CAD build for the part. Positions are in the model's coordinates, mm. Round coordinates to 2 decimals unless told otherwise and drop trailing zeros. Loops run counter-clockwise (first coordinate to the right, second up) from the corner with the lowest first, then second, coordinate; pieces in that order, holes last. Notation, with made-up numbers: (-36.75, 74.25) - (-3.75, 74.25) arc R18 ccw to (-3.75, 105.25) - close; hole circle Ø3 at (-21.75, 77). An arc over 180 degrees is marked (long way). Use one line per item in the form item = value.
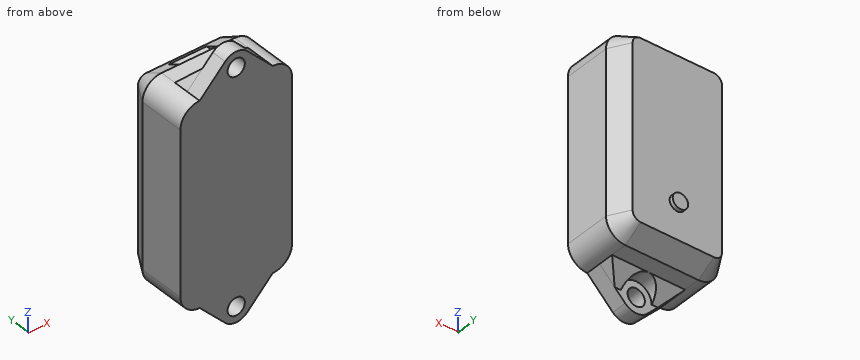
from build123d import *
from OCP.BRepFilletAPI import BRepFilletAPI_MakeChamfer

# Parameters (mm, degrees)
Y_KSEKLIK_EKSTR_ZYON2_DEPTH = 17.25
IZIM1_3_R                   = 2.25
Y_KSEKLIK_EKSTR_ZYON3_DEPTH = 4
PAH2_SIZE                   = 5
PAH2_SIZE2                  = 2.886751346
Y_KSEKLIK_EKSTR_ZYON4_DEPTH = 4
KES_EKSTR_ZYON2_DEPTH       = 24
IZIM7_W                     = 10
IZIM7_H                     = 2
KES_EKSTR_ZYON3_DEPTH       = 5
IZIM8_R                     = 2
Y_KSEKLIK_EKSTR_ZYON6_DEPTH = 1
IZIM10_R                    = 4
KES_EKSTR_ZYON4_DEPTH       = 10
IZIM11_R                    = 4
KES_EKSTR_ZYON5_DEPTH       = 10
KES_EKSTR_ZYON6_DEPTH       = 30


with BuildPart() as part:
    # izim1 → Y_kseklik-Ekstr_zyon2 (new body)
    with BuildSketch(Plane(origin=(0, 0, 0), x_dir=(1, 0, 0), z_dir=(0, 1, 0))):
        with BuildLine():
            Line((0, 26), (0, 5))
            ThreePointArc((0, 5), (1.464466094, 1.464466094), (5, 0))
            Line((5, 0), (24, 0))
            ThreePointArc((24, 0), (27.535533906, 1.464466094), (29, 5))
            Line((29, 5), (29, 26))
            Line((29, 26), (0, 26))
        make_face()
        with BuildLine():
            Line((0, 47), (0, 26))
            Line((0, 26), (29, 26))
            Line((29, 26), (29, 47))
            ThreePointArc((29, 47), (27.535533906, 50.535533906), (24, 52))
            Line((24, 52), (5, 52))
            ThreePointArc((5, 52), (1.464466094, 50.535533906), (0, 47))
        make_face()
    extrude(amount=Y_KSEKLIK_EKSTR_ZYON2_DEPTH)

    # izim1_3 → Y_kseklik-Ekstr_zyon3 (add)
    # profile 1 of 2: a face of its own
    with BuildSketch(Plane(origin=(0, 0, 0), x_dir=(1, 0, 0), z_dir=(0, 1, 0))):
        with BuildLine():
            ThreePointArc((11.638823529, 58.795294118), (14.5, 60), (17.361176471, 58.795294118))
            Line((17.361176471, 58.795294118), (24, 52))
            Line((24, 52), (5, 52))
            Line((5, 52), (11.638823529, 58.795294118))
        make_face()
        with Locations(Location((14.5, 56, 0), (0, 0, 270))):
            Circle(IZIM1_3_R, mode=Mode.SUBTRACT)
    # profile 2 of 2: a face of its own
    with BuildSketch(Plane(origin=(0, 0, 0), x_dir=(1, 0, 0), z_dir=(0, 1, 0))):
        with BuildLine():
            Line((5, 0), (11.638823529, -6.795294118))
            ThreePointArc((11.638823529, -6.795294118), (14.5, -8), (17.361176471, -6.795294118))
            Line((17.361176471, -6.795294118), (24, 0))
            Line((24, 0), (5, 0))
        make_face()
        with Locations(Location((14.5, -4, 0), (0, 0, 270))):
            Circle(IZIM1_3_R, mode=Mode.SUBTRACT)
    extrude(amount=Y_KSEKLIK_EKSTR_ZYON3_DEPTH)

    # Pah2: one chamfer whose edges measure the first distance from different faces: ONE call of the kernel's chamfer builder (chamfer() names one face for all edges)
    pah2_edges_1 = [part.edges().sort_by_distance(p)[0] for p in [
        (27.535533906, 17.25, -50.535533906),
    ]]
    pah2_side_1 = [part.faces().sort_by_distance(p)[0] for p in [
        (27.535533906, 8.625, -50.535533906),
    ]]
    pah2_edges_2 = [part.edges().sort_by_distance(p)[0] for p in [
        (14.5, 17.25, -52),
    ]]
    pah2_side_2 = [part.faces().sort_by_distance(p)[0] for p in [
        (14.5, 10.625, -52),
    ]]
    pah2_edges_3 = [part.edges().sort_by_distance(p)[0] for p in [
        (1.464466094, 17.25, -50.535533906),
    ]]
    pah2_side_3 = [part.faces().sort_by_distance(p)[0] for p in [
        (1.464466094, 8.625, -50.535533906),
    ]]
    pah2_edges_4 = [part.edges().sort_by_distance(p)[0] for p in [
        (0, 17.25, -26),
    ]]
    pah2_side_4 = [part.faces().sort_by_distance(p)[0] for p in [
        (0, 8.625, -26),
    ]]
    pah2_edges_5 = [part.edges().sort_by_distance(p)[0] for p in [
        (1.464466094, 17.25, -1.464466094),
    ]]
    pah2_side_5 = [part.faces().sort_by_distance(p)[0] for p in [
        (1.464466094, 8.625, -1.464466094),
    ]]
    pah2_edges_6 = [part.edges().sort_by_distance(p)[0] for p in [
        (14.5, 17.25, 0),
    ]]
    pah2_side_6 = [part.faces().sort_by_distance(p)[0] for p in [
        (14.5, 10.625, 0),
    ]]
    pah2_edges_7 = [part.edges().sort_by_distance(p)[0] for p in [
        (27.535533906, 17.25, -1.464466094),
    ]]
    pah2_side_7 = [part.faces().sort_by_distance(p)[0] for p in [
        (27.535533906, 8.625, -1.464466094),
    ]]
    pah2_edges_8 = [part.edges().sort_by_distance(p)[0] for p in [
        (29, 17.25, -26),
    ]]
    pah2_side_8 = [part.faces().sort_by_distance(p)[0] for p in [
        (29, 8.625, -26),
    ]]
    pah2 = BRepFilletAPI_MakeChamfer(part.part.solid().wrapped)
    for e in pah2_edges_1:
        pah2.Add(PAH2_SIZE, PAH2_SIZE2, e.wrapped, pah2_side_1[0].wrapped)  # the first distance lies on this face
    for e in pah2_edges_2:
        pah2.Add(PAH2_SIZE, PAH2_SIZE2, e.wrapped, pah2_side_2[0].wrapped)  # the first distance lies on this face
    for e in pah2_edges_3:
        pah2.Add(PAH2_SIZE, PAH2_SIZE2, e.wrapped, pah2_side_3[0].wrapped)  # the first distance lies on this face
    for e in pah2_edges_4:
        pah2.Add(PAH2_SIZE, PAH2_SIZE2, e.wrapped, pah2_side_4[0].wrapped)  # the first distance lies on this face
    for e in pah2_edges_5:
        pah2.Add(PAH2_SIZE, PAH2_SIZE2, e.wrapped, pah2_side_5[0].wrapped)  # the first distance lies on this face
    for e in pah2_edges_6:
        pah2.Add(PAH2_SIZE, PAH2_SIZE2, e.wrapped, pah2_side_6[0].wrapped)  # the first distance lies on this face
    for e in pah2_edges_7:
        pah2.Add(PAH2_SIZE, PAH2_SIZE2, e.wrapped, pah2_side_7[0].wrapped)  # the first distance lies on this face
    for e in pah2_edges_8:
        pah2.Add(PAH2_SIZE, PAH2_SIZE2, e.wrapped, pah2_side_8[0].wrapped)  # the first distance lies on this face
    add(Compound.cast(pah2.Shape()), mode=Mode.REPLACE)

    # izim4 → Y_kseklik-Ekstr_zyon4 (add)
    with BuildSketch(Plane(origin=(0, 4, 0), x_dir=(1, 0, 0), z_dir=(0, 1, 0))):
        with BuildLine():
            Line((8.907894737, 56), (12.25, 56))
            ThreePointArc((12.25, 56), (14.5, 53.75), (16.75, 56))
            Line((16.75, 56), (20.092105263, 56))
            Line((20.092105263, 56), (24, 52))
            Line((24, 52), (5, 52))
            Line((5, 52), (8.907894737, 56))
        make_face()
        with BuildLine():
            Line((5, 0), (8.907894737, -4))
            Line((8.907894737, -4), (12.25, -4))
            ThreePointArc((12.25, -4), (14.5, -1.75), (16.75, -4))
            Line((16.75, -4), (20.092105263, -4))
            Line((20.092105263, -4), (24, 0))
            Line((24, 0), (5, 0))
        make_face()
    extrude(amount=Y_KSEKLIK_EKSTR_ZYON4_DEPTH)

    # izim5 → Kes-Ekstr_zyon2 (cut)
    with BuildSketch(Plane.ZY):
        Polygon((0, 8), (4, 4), (4, 8), align=None)
    extrude(amount=-KES_EKSTR_ZYON2_DEPTH, mode=Mode.SUBTRACT)

    # izim7 → Kes-Ekstr_zyon3 (cut)
    with BuildSketch(Plane(origin=(0, 17.25, 0), x_dir=(1, 0, 0), z_dir=(0, 1, 0))):
        with Locations((14.5, 1)):
            Rectangle(IZIM7_W, IZIM7_H)
    extrude(amount=-KES_EKSTR_ZYON3_DEPTH, mode=Mode.SUBTRACT)

    # izim8 → Y_kseklik-Ekstr_zyon6 (add)
    with BuildSketch(Plane(origin=(0, 17.25, 0), x_dir=(1, 0, 0), z_dir=(0, 1, 0))):
        with Locations(Location((14.5, 40, 0), (0, 0, 270))):
            Circle(IZIM8_R)
    extrude(amount=Y_KSEKLIK_EKSTR_ZYON6_DEPTH)

    # izim10 → Kes-Ekstr_zyon4 (cut)
    with BuildSketch(Plane(origin=(0, 4, 0), x_dir=(1, 0, 0), z_dir=(0, 1, 0))):
        with Locations((14.5, 56)):
            Circle(IZIM10_R)
    extrude(amount=KES_EKSTR_ZYON4_DEPTH, mode=Mode.SUBTRACT)

    # izim11 → Kes-Ekstr_zyon5 (cut)
    with BuildSketch(Plane(origin=(0, 4, 0), x_dir=(1, 0, 0), z_dir=(0, 1, 0))):
        with Locations((14.5, -4)):
            Circle(IZIM11_R)
    extrude(amount=KES_EKSTR_ZYON5_DEPTH, mode=Mode.SUBTRACT)

    # izim12 → Kes-Ekstr_zyon6 (cut)
    with BuildSketch(Plane.ZY):
        Polygon((-52, 8), (-56, 8), (-56, 4), align=None)
    extrude(amount=-KES_EKSTR_ZYON6_DEPTH, mode=Mode.SUBTRACT)


solid = part.part
1) Slice it at A-A (z = -40). Write the cut outline in (x, y), plus the area to 3 significant figures.
Report:
outline = (0, 0) - (29, 0) - (29, 12.25) - (26.11, 17.25) - (16.5, 17.25) - (16.5, 18.25) - (12.5, 18.25) - (12.5, 17.25) - (2.89, 17.25) - (0, 12.25) - close
area = 490 mm^2
2) Drill centre lines: probe 1 along X at (y, z) = (2.6, -56); probe 2 along Y at (x, z) = (24.5, -17); probe 3 along Z at (x, y) = (13.5, 2). Where is each one in solid material? Low to high.
Report:
probe_1 = 8.91 to 12.25, 16.75 to 20.09
probe_2 = 0 to 17.25
probe_3 = -59.87 to -58.02, -53.98 to 1.98, 6.02 to 7.87
3) Slice it at B-B (x = 15.5). Write the cut outline in (y, z), plus the area to 3 significant figures.
Report:
outline = (0, -59.87) - (4, -59.87) - (4, -58.02) - (0, -58.02) - close; (0, -53.98) - (4, -53.98) - (4, -52.13) - (7.87, -52.13) - (8, -52) - (12.25, -52) - (17.25, -49.11) - (17.25, -41.73) - (18.25, -41.73) - (18.25, -38.27) - (17.25, -38.27) - (17.25, -2.89) - (15.71, -2) - (12.25, -2) - (12.25, 0) - (8, 0) - (7.87, 0.13) - (4, 0.13) - (4, 1.98) - (0, 1.98) - close; (0, 6.02) - (4, 6.02) - (4, 7.87) - (0, 7.87) - close
area = 914 mm^2
4) Slice it at C-C (z = -55). Write the cut outline in (x, y), plus the area to 3 significant figures.
Report:
outline = (7.93, 0) - (12.48, 0) - (12.48, 4) - (10.63, 4) - (10.63, 5) - (7.93, 5) - close; (16.52, 0) - (21.07, 0) - (21.07, 5) - (18.37, 5) - (18.37, 4) - (16.52, 4) - close
area = 41.8 mm^2
5) Slice it at D-D (x = 7.75). Write the cut outline in (y, z), plus the area to 3 significant figures.
Report:
outline = (0, -54.81) - (5.19, -54.81) - (8, -52) - (12.25, -52) - (17.25, -49.11) - (17.25, -2.89) - (12.25, 0) - (8, 0) - (5.19, 2.81) - (0, 2.81) - close
area = 920 mm^2
6) Flat gauge pins, fed straight in: pin 1 (9 mm diameter, centred on x = 17, z = 5, fed in from +Y); pin 2 (0.6 mm diameter, centred on y = 14, z = -1.5, fed in from +X); pin 3 (6 mm diameter, centred on x = 25.5, y = 7.5, fed in from +Z); pin 4 (4 mm diameter, centred on x = 14.5, z = 4, fed in from +Y). Where does each tip first touch, or does it go through?
Report:
pin_1 = 7.5
pin_2 = 26.48
pin_3 = 1.4
pin_4 = through
